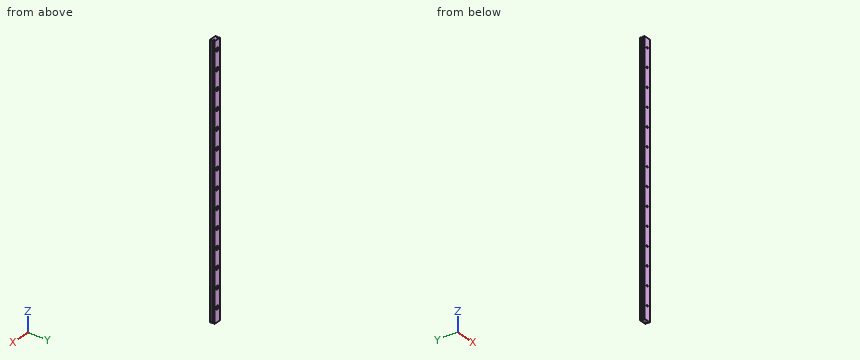
Autodesk Inventor part; units mm, degrees
ref_plane "YZ Plane" through (0, 0, 0) normal (1, 0, 0) x (0, 1, 0)
ref_plane "XZ Plane" through (0, 0, 0) normal (0, 1, 0) x (-1, 0, 0)
ref_plane "XY Plane" through (0, 0, 0) normal (0, 0, 1) x (1, 0, 0)
sketch "Skizze1" plane through (0, 0, 0) normal (0, 0, 1) x (1, 0, 0)
  line L0 (0, -1.9) -> (0, 11.4) construction
  line L1 (-7.5, 0) -> (7.5, 0)
  line L2 (7.5, 0) -> (7.5, 9.5)
  line L3 (7.5, 9.5) -> (-7.5, 9.5)
  line L4 (-7.5, 9.5) -> (-7.5, 0)
  circle A0 centre (-7.5, 6.5) radius 1.5
  line L5 (-12.6, 0) -> (12.6, 0)
  line L6 (-4.5, 6.5) -> (-7.5, 6.5) construction
  line L7 (-4.5, 7) -> (-7.5, 7)
  line L8 (-7.5, 6) -> (-4.5, 6)
  arc A1 (-4.5, 6) -> (-4.5, 7) centre (-4.5, 6.5) ccw
  arc A2 (-7.5, 7) -> (-7.5, 6) centre (-7.5, 6.5) ccw
  circle A3 centre (-4.5, 6.5) radius 1
  circle A4 centre (7.5, 6.5) radius 1.5
  line L9 (4.5, 7) -> (7.5, 7)
  line L10 (7.5, 6) -> (4.5, 6)
  arc A5 (4.5, 7) -> (4.5, 6) centre (4.5, 6.5) ccw
  circle A6 centre (4.5, 6.5) radius 1
  point P0 (0, 0)
  point P1 (0, 0)
  point P2 (-7.5, 8)
  point P3 (-7.5, 5)
  point P4 (-6, 6.5)
  point P5 (6, 6.5)
  point P6 (-6.0858, 7)
  point P7 (-5.366, 7)
  point P8 (-5.366, 6)
  point P9 (-6.0858, 6)
  point P10 (7.5, 5)
  point P11 (6.0858, 6)
  point P12 (5.366, 6)
  point P13 (5.366, 7)
  point P14 (6.0858, 7)
  point P15 (7.5, 8)
  dimension "d2" = 3
  dimension "d0" = 15
  dimension "d1" = 9.5
  dimension "d3" = 3
  dimension "d6" = 1
  dimension "d7" = 2
extrude "Extrusion1" add sketch "Skizze1" along normal blind 570 contours L4 A0 L8 A3 L7 L3 L2 A4 L9 A6 L10 L1
sketch "Skizze2" plane through (-7.5, 9.5, 570) normal (0, 1, 0) x (1, 0, 0)
  line L0 (-3, 570) -> (18, 570)
  line L1 (7.5, 688.8) -> (7.5, -114.8)
  circle A0 centre (7.5, 540) radius 3
  circle A1 centre (7.5, 540) radius 1.75
  point P0 (7.5, 570)
  dimension "d8" = 6
  dimension "d9" = 3.5
  dimension "d10" = 30
extrude "Extrusion2" cut sketch "Skizze2" against normal blind 6
extrude "Extrusion3" cut sketch "Skizze2" against normal blind 15 contours A1 L1 | L1 A1
chamfer "Fase1" distance 1 angle 45 1 edges at (-3, 9.5, 30)
pattern_linear "Rechteckige Anordnung1" count 14 spacing 40 along (0, 0, 1) of "Extrusion2", "Extrusion3", "Fase1"
equation "\"d4\" = Raillänge"
equation "\"Raillänge\" = 570"
properties part number "MGN15 Linear Rail 576mm"
Read the model definition and answer for the solid it produces. Units are mm, in the model's axes. Give positions to 0.01 mm unless a question says otherwise; leave off trailing zeros. Write each loop counter-clockwise with the first axis right and the second up, starting at its lowest first coordinate (ties: lowest second). Pieces come first, ordered by that corner, then holes. Notation, with made-up numbers: (-17.75, 4) - (-2.75, 4) arc R10 cw to (-2.75, 8) - close; hole circle Ø5 at (10, 17.5). An arc over 180 degrees is marked (long way). Use CSV: the item, a comma, the result in double quotes. Start each with the question number.
(1) Given P1, Ø2, axis at x = -5, y = 4.5, coming from the -Z side; P2, Ø4, axis at x = 0, z = 430, coming from the +Y side; P3, Ø7, axis at x = 0, z = 550, coming from the +Y side, each flat-ended and moving along its own axis, determine where each tip first touches the part or whether it passes through.
(2) Find section A-A (z = 210.5). Give the vertices of the cut face in (x, y).
(3) Consider line 1 along X through (y, z) = (6.7, 390); line 2 along Y through (x, z) = (4.75, 258); line 3 along X through (y, z) = (2.3, 350). Determine where each line is inside the solid, lowest interval first.
Findings below:
1,P1,"z = 0"
1,P2,"y = 3.5"
1,P3,"y = 9"
2,outline,"(-7.5, 0) - (7.5, 0) - (7.5, 5) arc R1.5 cw to (6.09, 6) - (5.37, 6) arc R1 cw (long way) to (5.37, 7) - (6.09, 7) arc R1.5 cw to (7.5, 8) - (7.5, 9.5) - (-7.5, 9.5) - (-7.5, 8) arc R1.5 cw to (-6.09, 7) - (-5.37, 7) arc R1 cw (long way) to (-5.37, 6) - (-6.09, 6) arc R1.5 cw to (-7.5, 5) - close"
3,line 1,"-3.52 to -3, 3 to 3.52"
3,line 2,"0 to 5.53, 7.47 to 9.5"
3,line 3,"-7.5 to -1.75, 1.75 to 7.5"
